Autodesk Inventor part; units mm, degrees
ref_plane "YZ Plane" through (0, 0, 0) normal (1, 0, 0) x (0, 1, 0)
ref_plane "XZ Plane" through (0, 0, 0) normal (0, 1, 0) x (-1, 0, 0)
ref_plane "XY Plane" through (0, 0, 0) normal (0, 0, 1) x (1, 0, 0)
sketch "Sketch1" plane through (0, 0, 0) normal (0, 1, 0) x (-1, 0, 0)
  line L0 (0, 0) -> (10, 0)
  line L1 (10, 0) -> (10, -60)
  line L2 (10, -60) -> (0, -60)
  line L3 (0, -60) -> (0, 0)
  line L4 (5, 0) -> (5, -6.25)
  circle A0 centre (5, -6.25) radius 1.3
  line L5 (5, -60) -> (5, -53.75)
  circle A1 centre (5, -53.75) radius 1.3
  dimension "d0" = 10
  dimension "d1" = 60
  dimension "d2" = 6.25
  dimension "d3" = 2.6
  dimension "d4" = 6.25
  dimension "d5" = 2.6
extrude "Extrusion1" add sketch "Sketch1" along normal blind 10
sketch "Sketch4" plane through (0, 10, 0) normal (0, 1, 0) x (1, 0, 0)
  line L0 (0, 0) -> (0, 60)
  line L1 (0, 0) -> (0, 10)
  line L2 (0, 60) -> (0, 40)
  line L3 (-10, 60) -> (-10, 0)
  line L4 (-10, 10) -> (-10, 50)
  line L5 (0, 50) -> (0, 10)
  line L6 (-10, 0) -> (0, 0)
  line L7 (0, 0) -> (0, 20)
  line L8 (0, 20) -> (-10, 20)
  line L9 (-10, 60) -> (-10, 40)
  line L10 (-10, 60) -> (10, 60) construction
  line L11 (-10, 40) -> (0, 40)
  dimension "d19" = 20
  dimension "d20" = 20
  dimension "d21" = 90
extrude "Extrusion3" cut sketch "Sketch4" against normal blind 5 contours L8 L3 L11 L0
sketch "Sketch8" plane through (0, 0, 0) normal (1, 0, 0) x (0, 0, -1)
  line L0 (40, 5) -> (20, 5)
  line L1 (20, 5) -> (20, 0)
  line L2 (40, 5) -> (40, 0)
  line L3 (60, 0) -> (0, 0)
extrude "Extrusion5" add sketch "Sketch8" along normal blind 15
sketch "Sketch9" plane through (0, 5, 0) normal (0, 1, 0) x (1, 0, 0)
  line L0 (15, 40) -> (15, 20)
  line L1 (15, 30) -> (11.5, 30)
  circle A0 centre (11.5, 30) radius 1.75
  point P0 (0, 0)
  dimension "d24" = 3.5
  dimension "d25" = 3.5
extrude "Extrusion6" cut sketch "Sketch9" against normal blind 5
properties part number "clawstack"
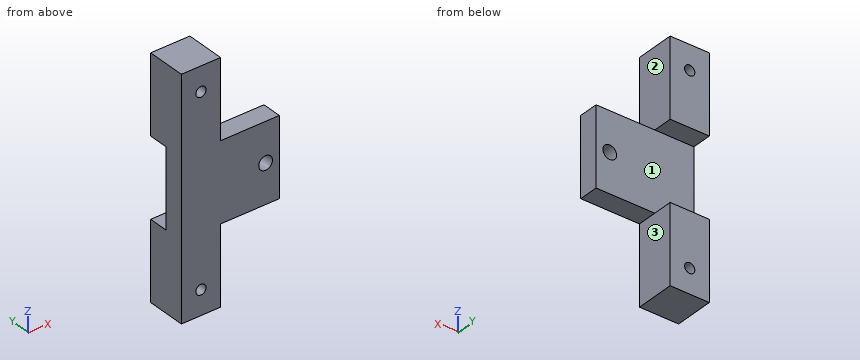
Work out the finished part from the listing and answer in its coordinate system (mm). Face numbers are marked on the shaded views. A direction names the side the tool comes from. Round coordinates to 2 decimals unless told otherwise and drop trailing zeros. Write each loop counter-clockwise with the first axis right and the second up, starting at its lowest first coordinate (ties: lowest second). Pieces come first, ordered by that corner, then holes.
1) A tool of negligible diameter and unlimited length cuts with its end or side. For the marked faces 1, 2 and 3, from which of +Z, -Z, +X, -X, +Y, -Y can it reach the whole face along a straight path? Write none if from no direction.
2) A cutting plane is placed at D-D (z = -53.75). Give the vertices of the cut face in (x, y).
3) Straight lines are drawn through the part: line 1 (Z direction, x = -5, y = 6); line 2 (Z direction, x = -5, y = 3); line 3 (X direction, y = 4.5, z = -6.25). For each, find the intervals that lie inside material, in ascending order.
4) A cutting plane is placed at B-B (x = -5). Give the vertices of the cut face in (y, z), plus the area to 3 significant figures.
5) A cutting plane is placed at A-A (y = 7.75). Give the vertices of the cut face in (x, z).
6) Given pin 1 Ø1.5 at (x, y) = (8, 2) entering from -Z; pin 2 Ø3 at (x, z) = (11, -26) entering from +Y; pin 3 Ø5 at (y, z) = (4.5, -9) entering from +X; pin 4 Ø5 at (x, y) = (6.5, 8.5) entering from -Z, each flat-ended and moving along its own axis, determine where each tip first touches the part or whether it passes through.
7) A cutting plane is placed at C-C (x = 11.5). Give the vertices of the cut face in (y, z), plus the area to 3 significant figures.
Completed:
1. face 1: +X, -X, +Y
1. face 2: +Z, +X, +Y, -Y
1. face 3: -Z, +X, +Y, -Y
2. outline: (-10, 0) - (-6.3, 0) - (-6.3, 10) - (-10, 10) - close; (-3.7, 0) - (0, 0) - (0, 10) - (-3.7, 10) - close
3. line 1: z = -60 to -55.05, -52.45 to -40, -20 to -7.55, -4.95 to 0
3. line 2: z = -60 to -55.05, -52.45 to -7.55, -4.95 to 0
3. line 3: x = -10 to -6.3, -3.7 to 0
4. outline: (0, -60) - (10, -60) - (10, -55.05) - (0, -55.05) - close; (0, -52.45) - (10, -52.45) - (10, -40) - (5, -40) - (5, -20) - (10, -20) - (10, -7.55) - (0, -7.55) - close; (0, -4.95) - (10, -4.95) - (10, 0) - (0, 0) - close
4. area: 448 mm2
5. outline: (-10, -60) - (0, -60) - (0, -40) - (-10, -40) - close; (-10, -20) - (0, -20) - (0, 0) - (-10, 0) - close; hole circle Ø2.6 at (-5, -53.75); hole circle Ø2.6 at (-5, -6.25)
6. pin 1: stops at z = -40
6. pin 2: stops at y = 5
6. pin 3: stops at x = 0
6. pin 4: passes through
7. outline: (0, -40) - (5, -40) - (5, -31.75) - (0, -31.75) - close; (0, -28.25) - (5, -28.25) - (5, -20) - (0, -20) - close
7. area: 82.5 mm2
